Can you work these out from the model? Positions are in its coordinate system, mm. A direction names the side the tool comes from. Give positions to 0.01 mm unless a question says otherwise; leave off trailing zeros. Write each loop counter-clockwise with the first axis right and the second up, starting at its lowest first coordinate (ties: lowest second). Pieces come first, ordered by that corner, then holes.
1. Suppose I cut it at A-A (x = 256). Please give me the cut outline in (y, z).
2. If I drill on probe 1 along X at (y, z) = (15, 31); probe 2 along X at (y, z) = (2.15, -53.34); probe 3 along Z at (x, y) = (-273.5, 2.5), over which ranges is the centre line in solid material (lowest first)?
3. Thinking about a two-plate mould opening in X: for faces 1 (the flat face through (-298.704, 14.3, -0.9)), 2 (the flat face through (295.656, 14.3, -0.9)), 3 (the flat face through (4, 0, -1)), which applies, pulls with the +X half, pulls with the -X half, needs draft (parallel to the pull), parting line crosses it, or undercut?
4. On a 3-axis mill with a long thin cutter (end or side, diameter ignored), from which of +Z, -Z, +X, -X, +Y, -Y can I reach the whole of each face in a straight line? I mean faces 4 (the flat face through (-295.656, 14.3, -0.9)), 5 (the flat face through (-1, 2, 63.5)). Say none if no direction works.
5. I'm going to push flat-ended pins straight in: pin 1 (1.5 mm diameter, centred on y = 2, z = 48.5, fed in from +X); pin 2 (2 mm diameter, centred on y = 2.5, z = -48, fed in from +X); pin 3 (10 mm diameter, centred on x = 164, z = -6, fed in from +Y). Where does each tip first touch, or does it pass through?
Autodesk Inventor part; units mm, degrees
ref_plane "YZ Plane" through (0, 0, 0) normal (1, 0, 0) x (0, 1, 0)
ref_plane "XZ Plane" through (0, 0, 0) normal (0, 1, 0) x (-1, 0, 0)
ref_plane "XY Plane" through (0, 0, 0) normal (0, 0, 1) x (1, 0, 0)
sketch "Sketch2" plane through (0, 0, 0) normal (0, 1, 0) x (-1, 0, 0)
  line L0 (-292.481, 63.5) -> (292.481, 63.5)
  line L1 (292.481, 63.5) -> (292.481, -63.5)
  line L2 (292.481, -63.5) -> (-292.481, -63.5)
  line L3 (-292.481, -63.5) -> (-292.481, 63.5)
  point P0 (0, 0)
  dimension "d0" = 292.481
  dimension "d1" = 292.481
  dimension "d2" = 63.5
  dimension "d3" = 63.5
extrude "Plate1" add sketch "Sketch2" along normal blind 3.048
sketch "Sketch3" plane through (-292.481, 0, 63.5) normal (0, 0, 1) x (1, 0, 0)
  arc A0 (584.962, 0) -> (591.185, 6.223) centre (584.962, 6.223) ccw
  line L0 (584.962, 6.223) -> (591.185, 6.223) construction
  line L1 (584.962, 6.223) -> (584.962, 0) construction
  line L2 (591.185, 6.223) -> (591.185, 19.5834)
  point P0 (584.962, 3.048)
  point P1 (292.481, 0)
  dimension "d5" = 90
  dimension "d6" = 6.223
  dimension "d7" = 6.223
  dimension "d8" = 13.3604
contour flange "Contour Flange1" sketch "Sketch3" thickness 3.048 bend radius 3.048 curves A0 L2 edges at (292.481, 0, 0) running between points at (292.481, 0, -63.5) (292.481, 0, 63.5)
bend "Bend1"
corner "Corner1"
sketch "Sketch4" plane through (-292.481, 0, 63.5) normal (0, 0, 1) x (1, 0, 0)
  arc A0 (-6.223, 6.223) -> (0, 0) centre (0, 6.223) ccw
  line L0 (0, 6.223) -> (-6.223, 6.223) construction
  line L1 (0, 6.223) -> (0, 0) construction
  line L2 (-6.223, 6.223) -> (-6.223, 19.5834)
  point P0 (0, 3.048)
  point P1 (292.481, 0)
  dimension "d18" = 90
  dimension "d19" = 6.223
  dimension "d20" = 6.223
  dimension "d21" = 13.3604
contour flange "Contour Flange2" sketch "Sketch4" thickness 3.048 bend radius 3.048 curves A0 L2 edges at (-292.481, 0, 0) running between points at (-292.481, 0, 63.5) (-292.481, 0, -63.5)
bend "Bend2"
corner "Corner2"
sketch "Sketch5" plane through (298.704, 6.223, -63.5) normal (1, 0, 0) x (0, 0, -1)
  line L0 (-127, 0) -> (-127, 13.3604)
  line L1 (0, -6.223) -> (-127, -6.223)
  point P0 (-63.5, -6.223)
  point P1 (-114.3, 6.477)
  dimension "d31" = 12.7
  dimension "d32" = 12.7
hole "Hole1" at (298.704, 12.7, 50.8) direction (-1, 0, 0) diameter 3.175 end through all
sketch "Sketch6" plane through (298.704, 6.223, -63.5) normal (1, 0, 0) x (0, 0, -1)
  circle A0 centre (-114.3, 6.477) radius 1.5875
  line L0 (-127, 0) -> (-127, 13.3604)
  line L1 (-114.3, 6.477) -> (-99.9256, 6.477)
  point P0 (-63.5, -6.223)
pattern_linear "Rectangular Pattern1" count 9 spacing 12.7 along (0, 0, -1) of "Hole1"
sketch "Sketch7" plane through (0, 3.048, 0) normal (0, 1, 0) x (1, 0, 0)
  line L0 (292.481, -63.5) -> (-292.481, -63.5)
  line L1 (-292.481, 63.5) -> (292.481, 63.5)
  line L2 (298.704, 63.5) -> (298.704, -63.5)
  line L3 (-298.704, -63.5) -> (-298.704, 63.5)
  point P0 (0, 0)
  point P1 (272.0086, -53.34)
  point P2 (272.0086, 53.34)
  point P3 (-272.0086, -53.34)
  point P4 (-272.0086, 53.34)
  point P5 (-272.0086, 31.3944)
  point P6 (-272.0086, -31.3944)
  point P7 (272.0086, -31.3944)
  point P8 (272.0086, 31.3944)
  point P9 (-212.725, -53.34)
  point P10 (-212.725, -31.3944)
  point P11 (-212.725, 31.3944)
  point P12 (-212.725, 53.34)
  point P13 (212.725, -53.34)
  point P14 (212.725, -31.3944)
  point P15 (212.725, 31.3944)
  point P16 (212.725, 53.34)
  dimension "d43" = 26.6954
  dimension "d44" = 10.16
  dimension "d45" = 10.16
  dimension "d46" = 26.6954
  dimension "d54" = 84.7344
  dimension "d55" = 84.7344
  dimension "d56" = 59.2836
  dimension "d57" = 59.2836
hole "Hole3" at (272.0086, 3.048, 53.34) at (272.0086, 3.048, -53.34) at (-272.0086, 3.048, 53.34) at (-272.0086, 3.048, -53.34) at (-272.0086, 3.048, -31.3944) at (-272.0086, 3.048, 31.3944) at (272.0086, 3.048, 31.3944) at (272.0086, 3.048, -31.3944) at (-212.725, 3.048, 53.34) at (-212.725, 3.048, 31.3944) at (-212.725, 3.048, -31.3944) at (-212.725, 3.048, -53.34) at (212.725, 3.048, 53.34) at (212.725, 3.048, 31.3944) at (212.725, 3.048, -31.3944) at (212.725, 3.048, -53.34) direction (0, -1, 0) diameter 8.382 end through all
equation "\"d38\" = Thickness"
equation "\"d63\" = Thickness"
equation "\"d9\" = BendReliefWidth"
equation "\"d10\" = BendReliefDepth"
equation "\"d11\" = MinimumRemnant"
equation "\"d12\" = BendRadius"
equation "\"d13\" = BendRadius"
equation "\"d15\" = CornerReliefSize"
equation "\"d16\" = GapSize"
equation "\"d17\" = JacobiRadiusSize"
equation "\"d22\" = BendReliefWidth"
equation "\"d23\" = BendReliefDepth"
equation "\"d24\" = MinimumRemnant"
equation "\"d25\" = BendRadius"
equation "\"d26\" = BendRadius"
equation "\"d28\" = CornerReliefSize"
equation "\"d29\" = GapSize"
equation "\"d30\" = JacobiRadiusSize"
equation "\"BendRadius\" = Thickness"
equation "\"BendReliefWidth\" = Thickness"
equation "\"BendReliefDepth\" = 0.5 * Thickness"
equation "\"CornerReliefSize\" = 4 * Thickness"
equation "\"MinimumRemnant\" = 2 * Thickness"
equation "\"TransitionRadius\" = BendRadius"
equation "\"JacobiRadiusSize\" = BendRadius"
equation "\"GapSize\" = Thickness"
equation "\"d4\" = BendRadius"
properties part number "Base Crossbar"
Checks:
1. outline: (0, -63.5) - (3.05, -63.5) - (3.05, 63.5) - (0, 63.5) - close
2. probe 1: x = -298.7 to -295.66, 295.66 to 298.7
2. probe 2: x = -297.19 to -276.2, -267.82 to -216.92, -208.53 to 208.53, 216.92 to 267.82, 276.2 to 297.19
2. probe 3: z = -63.5 to -57.26, -49.42 to -35.31, -27.48 to 27.48, 35.31 to 49.42, 57.26 to 63.5
3. face 1: pulls with the -X half
3. face 2: undercut
3. face 3: needs draft
4. face 4: +Z, -Z, +Y
4. face 5: +Z, +X, -X, +Y, -Y
5. pin 1: stops at x = 297.64
5. pin 2: stops at x = 298.08
5. pin 3: stops at y = 3.05
